Verification items for the finished model (mm, model axes). A direction names the side the tool comes from. Coordinates: 2 decimals unless noted, no trailing zeros. Order: outer loops, then holes, each group sorted by start corner. A loop starts at its lowest first (then second) coordinate and runs counter-clockwise, first axis right, second up. Notation, with made-up numbers: (-34, -25.5) -> (-30, -25.5) arc R20 cw to (-30, 1.5) -> close; hole circle Ø6 at (25, 1.25). An arc over 180 degrees is marked (long way). Write item = value, one per line. Start each with the question number.
1. Thickness scan on line 1 along X through (y, z) = (1.5, 0); line 2 along X through (y, z) = (1, 2.5); line 3 along Z through (x, y) = (-2.25, 1). Record the ranges inside material, lowest first. Write a range as from..to.
2. Release check for a two-part mould opening along Z. For faces 4 (the flat face through (-3, 0, 1.5)), 5 (the cylindrical face through (-1.775, 3.233, -1.341)), 6 (the flat face through (-4, 1.3, -1.3)) record: +Z half, -Z half, draft (parallel to the pull), parting line (faces both ways), or undercut.
3. Cross-section at A-A on x = 8. Record the cut outline in (y, z), plus the area to 3 significant figures.
4. Set-up check for faces 1 (the flat face through (-3.014, -1.293, 0.76)), 2 (the cylindrical face through (6, 0, -2)), 3 (the flat face through (12, 0, 0)): record each of +Z, -Z, +X, -X, +Y, -Y from which the full face is reachable in a straight line by a thin tool's end or side.
5. Go/stop test with flat-tipped pins: P1, Ø1, axis at x = -2.5, y = 1.5, coming from the +Z side; P2, Ø3, axis at x = 6, z = -1, coming from the +Y side; P3, Ø0.5, axis at x = -3, y = 0.5, coming from the +Z side. Record where each tip stops, or that it passes through.
Autodesk Inventor part; units mm, degrees
ref_plane "SCW_XY" through (0, 0, 0) normal (1, 0, 0) x (0, 0, -1)
ref_plane "SCW_YZ" through (0, 0, 0) normal (0, 0, -1) x (0, 1, 0)
ref_plane "SCW_ZX" through (0, 0, 0) normal (0, 1, 0) x (1, 0, 0)
sketch "Sketch_1" plane through (0, 0, 0) normal (0, 0, 1) x (1, 0, 0)
  line L0 (12, 0) -> (-4, 0)
  line L1 (-4, 0) -> (-4, 3.1)
  line L2 (-4, 3.1) -> (-3.6, 3.5)
  line L3 (-3.6, 3.5) -> (0, 3.5)
  line L4 (0, 3.5) -> (0, 2.2)
  arc A0 (0, 2.2) -> (0.2, 2) centre (0.2, 2.2) ccw
  line L5 (0.2, 2) -> (11.5705, 2)
  line L6 (11.5705, 2) -> (12, 1.5705)
  line L7 (12, 1.5705) -> (12, 0)
  line L8 (12, 0) -> (-4, 0)
revolve "Revolution1" add sketch "Sketch_1" angle 360 about axis through (12, 0, 0) along (1, 0, 0)
thread "Thread1"
sketch "Sketch_2" plane through (-4, 0, 0) normal (1, 0, 0) x (0, 0, -1)
  line L0 (-1.5, -0.866) -> (0, -1.7321)
  line L1 (0, -1.7321) -> (1.5, -0.866)
  line L2 (1.5, -0.866) -> (1.5, 0.866)
  line L3 (1.5, 0.866) -> (0, 1.7321)
  line L4 (0, 1.7321) -> (-1.5, 0.866)
  line L5 (-1.5, 0.866) -> (-1.5, -0.866)
extrude "Extrusion1" cut sketch "Sketch_2" along normal blind 2
sketch "Sketch_5" plane through (0, 0, 0) normal (0, 0, 1) x (1, 0, 0)
  line L0 (-1.134, 0) -> (-2, 0)
  line L1 (-2, 0) -> (-2, 1.5)
  line L2 (-2, 1.5) -> (-1.134, 0)
  line L3 (-1.134, 0) -> (-2, 0)
revolve "Revolution2" cut sketch "Sketch_5" angle 360 about axis through (-1.134, 0, 0) along (1, 0, 0)
ref_plane "SCW_XY" through (0, 0, 0) normal (1, 0, 0) x (0, 0, -1)
ref_plane "SCW_YZ" through (0, 0, 0) normal (0, 0, -1) x (0, 1, 0)
ref_plane "SCW_ZX" through (0, 0, 0) normal (0, 1, 0) x (1, 0, 0)
properties part number "M4-12_bo2"
Worked out:
q1.line_1 = -2..12
q1.line_2 = -4..0
q1.line_3 = -3.35..-1.27, 1.27..3.35
q2.face_4 = undercut
q2.face_5 = parting line
q2.face_6 = draft
q3.outline = circle Ø4 at (0, 0)
q3.area = 12.6 mm²
q4.face_1 = -X
q4.face_2 = +X
q4.face_3 = +Z, -Z, +X, +Y, -Y
q5.P1 = 3.35
q5.P2 = 2
q5.P3 = 3.49
